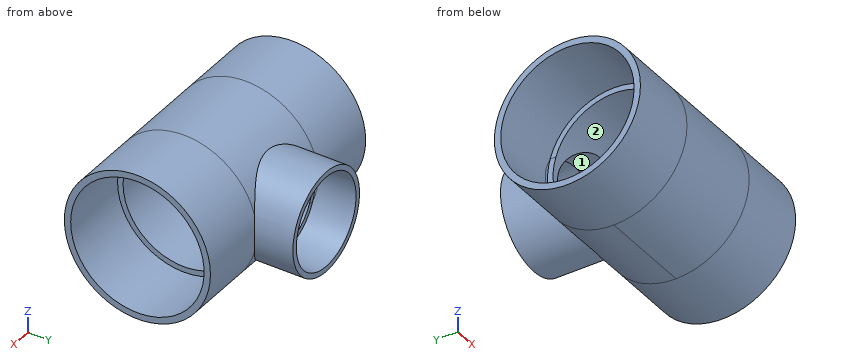
from build123d import *

# Parameters (mm, degrees)
SKETCH4_R           = 92.456
BOSS_EXTRUDE1_DEPTH = 119.38
SKETCH5_R           = 64.008
BOSS_EXTRUDE2_DEPTH = 89.408


with BuildPart() as part:
    # Sketch1 → Revolve1 (revolve)
    with BuildSketch(Plane.XY):
        Polygon((-149.098, -92.456), (-59.69, -92.456), (-59.69, -83.9978), (-149.098, -84.4169), align=None)
        Polygon((149.098, -84.4169), (59.69, -83.9978), (59.69, -92.456), (149.098, -92.456), align=None)
    revolve(axis=Axis((-149.098, 0, 0), (1, 0, 0)))



with BuildPart() as body_2:
    # Sketch2 → Revolve2 (revolve)
    with BuildSketch(Plane.XY):
        Polygon((57.3786, 140.716), (57.0357, 89.408), (64.008, 89.408), (64.008, 140.716), align=None)
    revolve(axis=Axis((0, 0, 0), (0, 1, 0)))


with BuildPart() as part_1:
    add(part.part)

    add(body_2.part)  # Boss-Extrude1 merges body 2
    # Sketch4 → Boss-Extrude1 (add)
    with BuildSketch(Plane(origin=(-59.69, 0, 0), x_dir=(0, 0, -1), z_dir=(1, 0, 0))):
        Circle(SKETCH4_R)
    extrude(amount=BOSS_EXTRUDE1_DEPTH)

    # Sketch5 → Boss-Extrude2 (add)
    with BuildSketch(Plane.XZ.offset(-89.408)):
        Circle(SKETCH5_R)
    extrude(amount=BOSS_EXTRUDE2_DEPTH)

    # Sketch6 → Cut-Revolve1 (revolve, cut)
    with BuildSketch(Plane.XY):
        Polygon((-149.098, -84.4169), (-59.69, -83.9978), (-59.69, -77.0255), (59.69, -77.0255), (59.69, -83.9978), (149.098, -84.4169), (149.098, 0), (-149.098, 0), align=None)
    revolve(axis=Axis((149.098, 0, 0), (-1, 0, 0)), mode=Mode.SUBTRACT)

    # Sketch7 → Cut-Revolve2 (revolve, cut)
    with BuildSketch(Plane.XY):
        Polygon((57.3786, 140.716), (57.0357, 89.408), (51.1302, 89.408), (51.1302, 0), (0, 0), (0, 140.716), align=None)
    revolve(axis=Axis((0, 0, 0), (0, 1, 0)), mode=Mode.SUBTRACT)


solid = part_1.part
The model under review builds one solid part; all positions refer to its coordinate system, in mm. Face numbers are marked on the shaded views. A direction names the side the tool comes from. Coordinates: 2 decimals unless noted, no trailing zeros. Loops run counter-clockwise (first coordinate to the right, second up) from the corner with the lowest first, then second, coordinate; pieces in that order, holes last. Notation, with made-up numbers: M 70,-17.5 L 93,-17.5 A8 ccw 93,-4.5 Z; hole C -0.75,35 d1. An arc over 180 degrees is marked long. Put each result on its own line as item: value. Start each with the question number.
Q1. For the marked faces 1 and 2, list the 3-axis set-ups (+Z, -Z, +X, -X, +Y, -Y) from which the entire face can be reached by the end or side of a thin tool; tool diameter is ignored.
Q2. Clearance check with flat-ended pins moving along their axes: pin 1 (1 mm diameter, centred on x = 63.5, y = 47.5, fed in from +Z); pin 2 (6 mm diameter, centred on x = -19.5, z = -40.5, fed in from +Y); pin 3 (4 mm diameter, centred on x = 58, y = 52, fed in from +Z); pin 4 (9.5 mm diameter, centred on x = 52.5, z = 10, fed in from +Y). State where each tip first meets the part, or that it passes through.
Q3. Add section B-B (x = -89). Write out the cut boundary in (y, z), and give its area (3 significant figures).
Q4. Wall thickness on line 1 (Z direction, x = 0, y = 67.5); line 2 (Z direction, x = 6.5, y = 0); line 3 (Y direction, x = 35, z = 0): over which ranges is each line inside the solid? List them lowest first.
Q5. Add section A-A (z = -6.5). Count the separate pieces of the cut face and the enclosed holes in it, and give its area (3 significant figures).
Answers:
1. face 1: +Y
1. face 2: +X, -X
2. pin 1: stops at z = 79.62
2. pin 2: stops at y = -63.57
2. pin 3: stops at z = 77.77
2. pin 4: stops at y = 140.72
3. outline: C 0,0 d184.91; hole C 0,0 d168.27
3. area: 4,620 mm^2
4. line 1: z = -64.01 to -51.13, 51.13 to 64.01
4. line 2: z = -92.46 to -77.03, 77.03 to 92.46
4. line 3: y = -92.46 to -77.03
5. separate pieces: 3
5. enclosed holes: 0
5. area: 5,710 mm^2
